Here's the drawing with two shaded views (mm, measured from the low corner). I have some questions. A direction names the side the tool comes from. Round coordinates to 2 decimals unless told otherwise and drop trailing zeros. Loops run counter-clockwise (first coordinate to the right, second up) from the corner with the lowest first, then second, coordinate; pieces in that order, holes last.
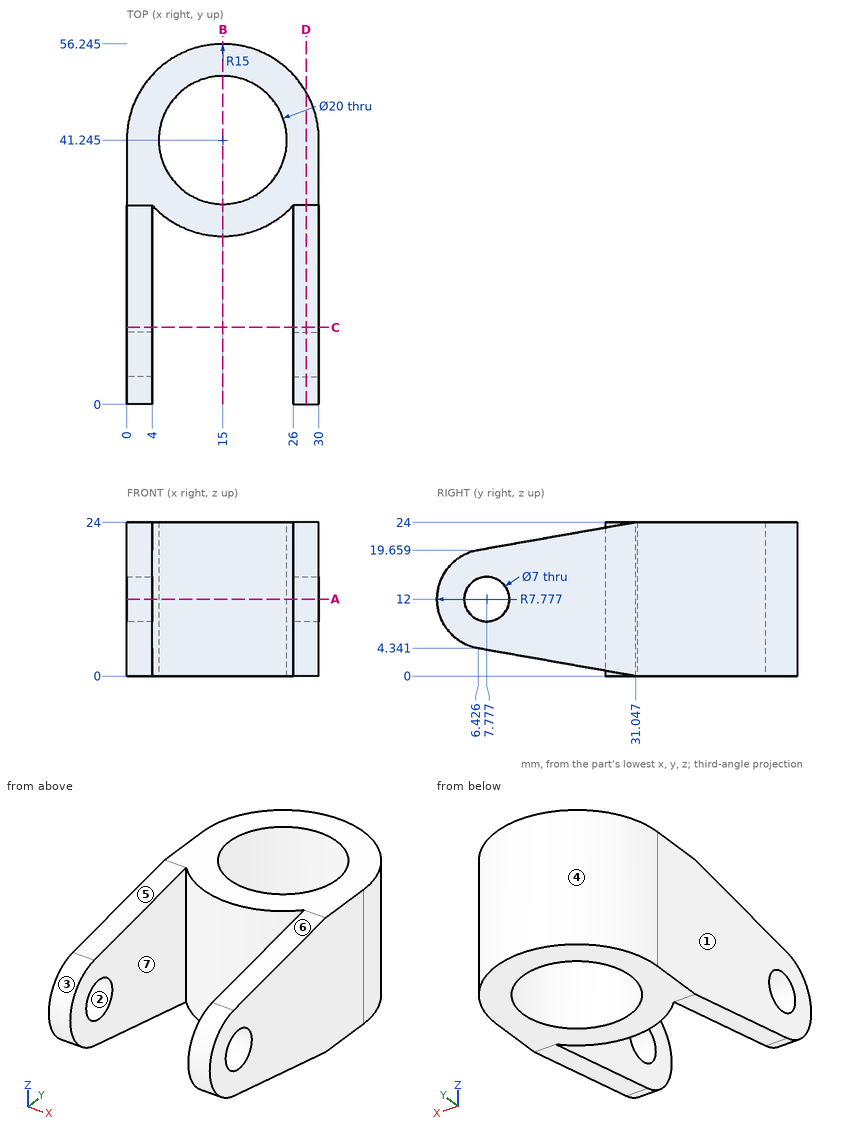
(1) If we section it at B-B, the plane x = 15: List the corners of the cut face in (y, z) for me (1 decimal).
Worked answers:
outline: (26.2, 0) - (31.2, 0) - (31.2, 24) - (26.2, 24) - close; (51.2, 0) - (56.2, 0) - (56.2, 24) - (51.2, 24) - close
(2) For the marked faces 5, 6 and 7, which set-ups out of +Z, -Z, +X, -X, +Y, -Y let a thin tool reach every point of the face, with its end or its side?
Worked answers:
face 5: +Z, -X, -Y
face 6: +Z, +X, -Y
face 7: +Z, -Z, -Y
(3) Will these pins go through, and if not, where does the flat tip stop? P1, Ø18, axis at x = 15, y = 41.24, coming from the +Z side; P2, Ø5, axis at x = 23.5, z = 4, coming from the +Y side; P3, Ø1.5, axis at x = 4.5, y = 7.5, coming from the +Z side.
Worked answers:
P1: passes through
P2: stops at y = 54.99
P3: stops at z = 19.95
(4) If we section it at C-C, the plane y = 12: List the corners of the cut face in (x, z) for me, then the cut area to 3 significant figures.
Worked answers:
outline: (0, 3.36) - (4, 3.36) - (4, 20.64) - (0, 20.64) - close; (26, 3.36) - (30, 3.36) - (30, 20.64) - (26, 20.64) - close
area: 138 mm2
(5) If we section it at D-D, the plane x = 28: List the corners of the cut face in (y, z) for me.
Worked answers:
outline: (6.43, 4.34) - (31.05, 0) - (48.73, 0) - (48.73, 24) - (31.05, 24) - (6.43, 19.66) arc R7.78 ccw to start; hole circle Ø7 at (7.78, 12)
(6) If we mould it in two halves opening along Y, with no side actions, what happens to the marked faces 1, 2, 3 and 4? For each: released by +Y, released by -Y, zero draft, split by the parting line, or undercut.
Worked answers:
face 1: zero draft
face 2: undercut
face 3: released by -Y
face 4: released by +Y
(7) If I drill on line 1 (X direction, y = 12, z = 17); line 2 (Y direction, x = 15, z = 11.25) (1 decimal); line 3 (X direction, y = 30, z = 16.5) (1 decimal), over which ranges is the centre line in solid material (lowest first)?
Worked answers:
line 1: x = 0 to 4, 26 to 30
line 2: y = 26.2 to 31.2, 51.2 to 56.2
line 3: x = 0 to 4, 5.1 to 24.9, 26 to 30
(8) If we section it at A-A, the plane z = 12: List the corners of the cut face in (x, y) for me (1 decimal).
Worked answers:
outline: (0, 0) - (4, 0) - (4, 4.3) - (0, 4.3) - close; (0, 11.3) - (4, 11.3) - (4, 31) arc R15 ccw to (26, 31) - (26, 11.3) - (30, 11.3) - (30, 41.2) arc R15 ccw to (0, 41.2) - close; (26, 0) - (30, 0) - (30, 4.3) - (26, 4.3) - close; hole circle Ø20 at (15, 41.2)
